from build123d import *

# Parameters (mm, degrees)
F0_W      = 23.749
F0_H      = 15.7988
F1_DEPTH  = 9.5504
F2_R      = 2.4511
F8_DEPTH  = 1.778
F4_R      = 2.4511
F9_DEPTH  = 1.778
F6_R      = 2.4511
F10_DEPTH = 1.778
F3_R      = 2.4511
F11_DEPTH = 1.778
F5_R      = 2.4511
F12_DEPTH = 1.778
F7_R      = 2.4511
F13_DEPTH = 1.778
F14_W     = 22.5298
F14_H     = 14.5796
F17_DEPTH = 8.3312
F15_R     = 3.2385
F18_DEPTH = 8.3312
F16_R     = 3.2385
F19_DEPTH = 8.3312
F20_R     = 2.794
F22_DEPTH = 8.3312
F21_R     = 2.794
F23_DEPTH = 8.3312


with BuildPart() as f1:
    # F0 (on Top) → F1 (new body)
    with BuildSketch(Plane.XY):
        Rectangle(F0_W, F0_H)
    extrude(amount=F1_DEPTH)

    # F2 (on face) → F8 (join)
    with BuildSketch(Plane.XY.offset(9.5504)):
        with Locations((-7.9502, 3.9751)):
            Circle(F2_R)
    extrude(amount=F8_DEPTH)

    # F4 (on face) → F9 (join)
    with BuildSketch(Plane.XY.offset(9.5504)):
        with Locations((7.9502, 3.9751)):
            Circle(F4_R)
    extrude(amount=F9_DEPTH)

    # F6 (on face) → F10 (join)
    with BuildSketch(Plane.XY.offset(9.5504)):
        with Locations((7.9502, -3.9751)):
            Circle(F6_R)
    extrude(amount=F10_DEPTH)

    # F3 (on face) → F11 (join)
    with BuildSketch(Plane.XY.offset(9.5504)):
        with Locations((0.0508, 3.975429)):
            Circle(F3_R)
    extrude(amount=F11_DEPTH)

    # F5 (on face) → F12 (join)
    with BuildSketch(Plane.XY.offset(9.5504)):
        with Locations((-7.9502, -3.9751)):
            Circle(F5_R)
    extrude(amount=F12_DEPTH)

    # F7 (on face) → F13 (join)
    with BuildSketch(Plane.XY.offset(9.5504)):
        with Locations((0.0254, -3.9751)):
            Circle(F7_R)
    extrude(amount=F13_DEPTH)

    # F14 (on face) → F17 (cut)
    with BuildSketch(Plane(origin=(0, 0, 0), x_dir=(1, 0, 0), z_dir=(0, 0, -1))):
        Rectangle(F14_W, F14_H)
    extrude(amount=-F17_DEPTH, mode=Mode.SUBTRACT)

    # F15 (on face) → F18 (join)
    with BuildSketch(Plane(origin=(0, 0, 0), x_dir=(1, 0, 0), z_dir=(0, 0, -1))):
        with Locations((-5.4102, -0.0127)):
            Circle(F15_R)
    extrude(amount=-F18_DEPTH)

    # F16 (on face) → F19 (join)
    with BuildSketch(Plane(origin=(0, 0, 0), x_dir=(1, 0, 0), z_dir=(0, 0, -1))):
        with Locations((5.4102, 0)):
            Circle(F16_R)
    extrude(amount=-F19_DEPTH)

    # F20 (on face) → F22 (cut)
    with BuildSketch(Plane(origin=(0, 0, 0), x_dir=(1, 0, 0), z_dir=(0, 0, -1))):
        with Locations((-5.4102, -0.0127)):
            Circle(F20_R)
    extrude(amount=-F22_DEPTH, mode=Mode.SUBTRACT)

    # F21 (on face) → F23 (cut)
    with BuildSketch(Plane(origin=(0, 0, 0), x_dir=(1, 0, 0), z_dir=(0, 0, -1))):
        with Locations((5.4102, 0)):
            Circle(F21_R)
    extrude(amount=-F23_DEPTH, mode=Mode.SUBTRACT)


solid = f1.part
Can you work these out from the model? Positions are in its coordinate system, mm. A direction names the side the tool comes from. Coordinates: 2 decimals unless noted, no trailing zeros. Order: outer loops, then holes, each group sorted by start corner. A loop starts at its lowest first (then second) coordinate and runs counter-clockwise, first axis right, second up. Notation, with made-up numbers: (54, 17) - (76, 17) arc R16 ccw to (76, 28) - close; hole circle Ø7 at (58, 0.25). An arc over 180 degrees is marked (long way). Answer as a JSON object with one key per item and string values. Group by question number.
Q1. Imagine slicing it at B-B (y = -6). Please give me the cut outline in (x, z).
Q2. Imagine slicing it at A-A (z = 5.5). Please give me the cut outline in (x, y).
Q3. Will these pins go through, and if not, where does the flat tip stop? P1, Ø1.5, axis at x = 1.5, y = 6, coming from the -Z side; P2, Ø9, axis at x = 5.41, y = 0, coming from the +Z side.
Q4. On a 3-axis mill with a long thin cutter (end or side, diameter ignored), from which of +Z, -Z, +X, -X, +Y, -Y can I reach the whole of each face in a straight line? I mean faces 3 (the face through (11.265, 0, 4)), 4 (the face through (-9.895, 2.484, 10.427)), 5 (the face through (-0.9, -7.6, 0)). Say none if no direction works.
Q5. I need wall thicknesses on line 1 (X direction, y = 0, z = 4.5); line 2 (Y direction, x = -5.25, z = 6); line 3 (X direction, y = 6.75, z = 8.25). Which ranges of each line are inside material? Lowest first, please. Write a range as from..to.
Q6. Imagine slicing it at D-D (z = 10.5). Please give me the cut outline in (x, y).
Q7. Imagine slicing it at C-C (x = -4.75). Please give me the cut outline in (y, z), and give its area (3 significant figures).
Q8. We'd pull the mould along Y, two halves only. Please class faces 1 (the face through (-7.797, -2.176, 4.107)), 2 (the face through (0, 4, 11.328)): +Y half, -Y half, draft (parallel to the pull), parting line (faces both ways), or undercut.
Determined:
{
 "1": {"outline": "(-11.87, 0) - (-11.26, 0) - (-11.26, 8.33) - (11.26, 8.33) - (11.26, 0) - (11.87, 0) - (11.87, 9.55) - (9.33, 9.55) - (9.33, 11.33) - (6.57, 11.33) - (6.57, 9.55) - (1.41, 9.55) - (1.41, 11.33) - (-1.36, 11.33) - (-1.36, 9.55) - (-6.57, 9.55) - (-6.57, 11.33) - (-9.33, 11.33) - (-9.33, 9.55) - (-11.87, 9.55) - close"},
 "2": {"outline": "(-11.87, -7.9) - (11.87, -7.9) - (11.87, 7.9) - (-11.87, 7.9) - close; circle Ø6.48 at (-5.41, 0.01); circle Ø6.48 at (5.41, 0); hole (-11.26, -7.29) - (11.26, -7.29) - (11.26, 7.29) - (-11.26, 7.29) - close; hole circle Ø5.59 at (-5.41, 0.01); hole circle Ø5.59 at (5.41, 0)"},
 "3": {"P1": "stops at z = 8.33", "P2": "stops at z = 11.33"},
 "4": {"face 3": "-Z", "face 4": "+Z", "face 5": "-Z, +X, -X, +Y, -Y"},
 "5": {"line 1": "x = -11.87..-11.26, -8.65..-8.2, -2.62..-2.17, 2.17..2.62, 8.2..8.65, 11.26..11.87", "line 2": "y = -7.9..-7.29, -3.22..-2.78, 2.8..3.25, 7.29..7.9", "line 3": "x = -11.87..-11.26, 11.26..11.87"},
 "6": {"outline": "circle Ø4.9 at (-7.95, -3.98); circle Ø4.9 at (-7.95, 3.98); circle Ø4.9 at (0.03, -3.98); circle Ø4.9 at (0.05, 3.98); circle Ø4.9 at (7.95, -3.98); circle Ø4.9 at (7.95, 3.98)"},
 "7": {"outline": "(-7.9, 0) - (-7.29, 0) - (-7.29, 8.33) - (-3.16, 8.33) - (-3.16, 0) - (-2.7, 0) - (-2.7, 8.33) - (2.73, 8.33) - (2.73, 0) - (3.18, 0) - (3.18, 8.33) - (7.29, 8.33) - (7.29, 0) - (7.9, 0) - (7.9, 9.55) - (-7.9, 9.55) - close", "area": "37.0 mm2"},
 "8": {"face 1": "undercut", "face 2": "draft"}
}
